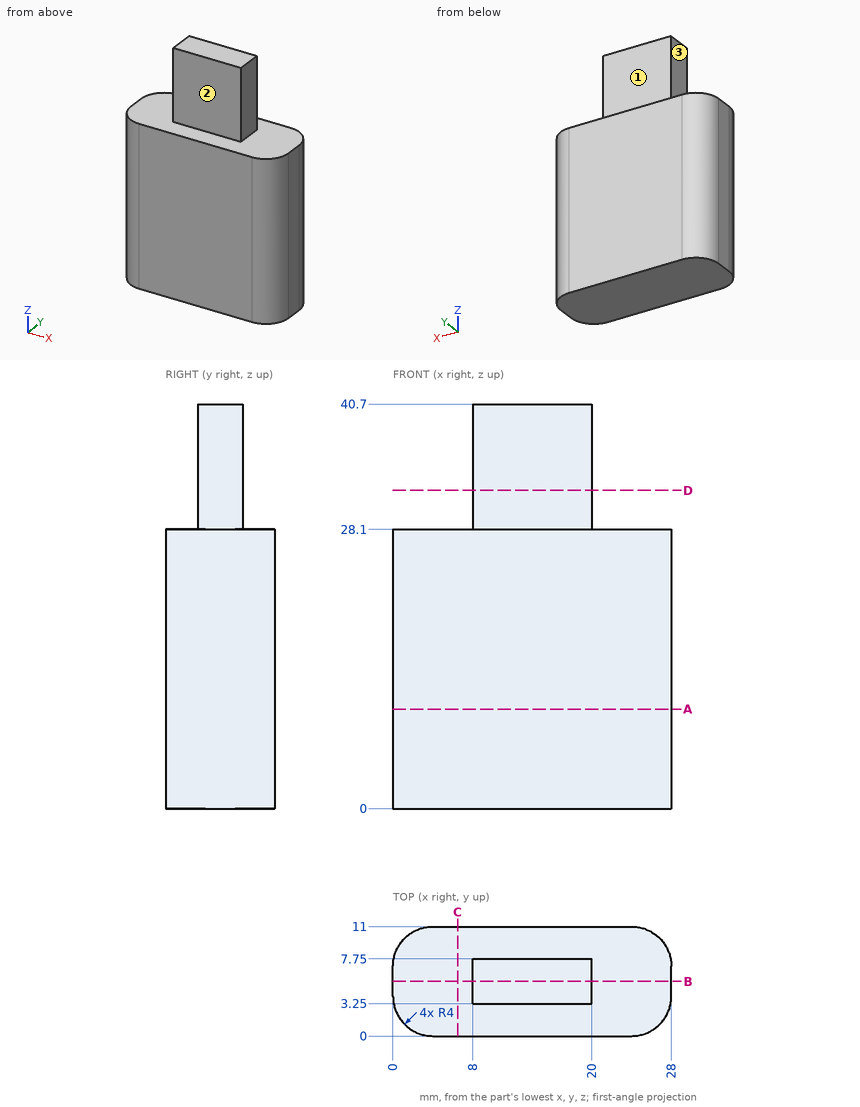
Design review of the part shown in the three views and the two pictorial views. Dimensions are in mm from the part's minimum x, y and z. A direction names the side the tool comes from. Coordinates: 2 decimals unless noted, no trailing zeros. Write each loop counter-clockwise with the first axis right and the second up, starting at its lowest first coordinate (ties: lowest second). Pieces come first, ordered by that corner, then holes.
(1) Tool access review of the marked faces 1, 2 and 3: name each direction out of +Z, -Z, +X, -X, +Y, -Y from which nothing blocks a thin tool from reaching the whole face with its end or side.
(2) Add section B-B on y = 5.5. Give the boundary of the cut face in (x, z), then the cut area to 3 significant figures.
(3) Add section A-A on z = 10. Give the boundary of the cut face in (x, y).
(4) Add section C-C on x = 6.5. Give the boundary of the cut face in (y, z), then the cut area to 3 significant figures.
(5) Wall thickness on probe 1 along Z at (x, y) = (4.75, 3); probe 2 along Y at (x, z) = (19.75, 31); probe 3 along X at (y, z) = (10, 24): over which ranges is each line inside the solid? List them lowest first.
(6) Add section D-D on z = 32. Give the boundary of the cut face in (x, y), then the cut area to 3 significant figures.
(7) For pin 1 Ø3.5 at (x, z) = (15.5, 37.5) entering from -Y; pin 2 Ø2 at (y, z) = (6.5, 32.5) entering from +X; pin 3 Ø9.5 at (x, z) = (14, 34.5) entering from +Y, all flat-tipped, find the tip position at first contact; note any pin that passes through.
Answer sheet:
1. face 1: +Z, +X, -X, +Y
1. face 2: +Z, +X, -X, -Y
1. face 3: +Z, -X, +Y, -Y
2. outline: (0, 0) - (28, 0) - (28, 28.1) - (20, 28.1) - (20, 40.7) - (8, 40.7) - (8, 28.1) - (0, 28.1) - close
2. area: 938 mm2
3. outline: (0, 4) arc R4 ccw to (4, 0) - (24, 0) arc R4 ccw to (28, 4) - (28, 7) arc R4 ccw to (24, 11) - (4, 11) arc R4 ccw to (0, 7) - close
4. outline: (0, 0) - (11, 0) - (11, 28.1) - (0, 28.1) - close
4. area: 309 mm2
5. probe 1: z = 0 to 28.1
5. probe 2: y = 3.25 to 7.75
5. probe 3: x = 1.35 to 26.65
6. outline: (8, 3.25) - (20, 3.25) - (20, 7.75) - (8, 7.75) - close
6. area: 54.0 mm2
7. pin 1: stops at y = 3.25
7. pin 2: stops at x = 20
7. pin 3: stops at y = 7.75
